from build123d import *

# Parameters (mm, degrees)
VERRUNDUNG1_R = 0.5


with BuildPart() as part:
    # Skizze1 → Rotation1 (revolve)
    with BuildSketch(Plane.XY, mode=Mode.PRIVATE) as rotation1_sk:
        Polygon((20, 0), (21.65, 0), (21.65, 0.5), (24.525, 0.5), (24.525, 0), (26, 0), (26, 7), (24.525, 7), (24.525, 6.5), (21.65, 6.5), (21.65, 7), (20, 7), align=None)
    revolve(rotation1_sk.sketch.rotate(Axis((0, 0, 0), (0, 1, 0)), 90), axis=Axis((0, 0, 0), (0, 1, 0)))

    # Verrundung1
    verrundung1_edges = [part.edges().sort_by_distance(p)[0] for p in [
        (0, 7, 26),
        (0, 0, 26),
        (0, 7, 20),
    ]]
    fillet(verrundung1_edges, radius=VERRUNDUNG1_R)


solid = part.part
Part model, mm, in its own coordinate system. A direction names the side the tool comes from. Coordinates: 2 decimals unless noted, no trailing zeros. Loops run counter-clockwise (first coordinate to the right, second up) from the corner with the lowest first, then second, coordinate; pieces in that order, holes last. Notation, with made-up numbers: (16, 62) -> (56, 62) arc R20 ccw to (56, 86) -> close; hole circle Ø11 at (16.25, -10.5). An arc over 180 degrees is marked (long way). Use a Markdown table: item, result. Add a question column.
Item 1: Which spindle directions (+Z, -Z, +X, -X, +Y, -Y) get a long thin tool onto all of the face, cutting with end or side? Do faces 1 (the flat face through (22, 6.5, 0)), 2 (the flat face through (19.1, 7, -7.9)), 3 (the cylindrical face through (21.758, 0.246, -11.317)). Say none if no direction does.
Item 2: Flat gauge pins, fed straight in: P1, Ø12, axis at x = 16, z = 18, coming from the +Y side; P2, Ø1.5, axis at x = 15, y = 6, coming from the -Z side; P3, Ø2, axis at y = 5.5, z = 0.5, coming from the +X side; P4, Ø3, axis at y = 4.5, z = 4.5, coming from the -X side. Where does each tip first touch, or does it go through?
Item 3: Band-saw the part on C-C on y = 5.75. Write the cut outline in (x, z).
Item 4: Pull direction Z, two halves, no side cores. Call faces 4 (the cylindrical face through (-0.88, 3.2, 19.98)), 5 (the cylindrical face through (15.821, 3.542, 20.633)), 6 (the flat face through (-13, 0, -21)): +Z half, -Z half, draft (parallel to the pull), parting line (faces both ways), or undercut.
Item 5: Probe probe 1 along X at (y, z) = (1.75, 0); probe 2 along Z at (x, y) = (0.5, 5.75); probe 3 along Y at (x, z) = (-20, 10). List the from-to ranges inside material, lowest first.
Geometry says:
| question | item | result |
|---|---|---|
| 1 | face 1 | +Y |
| 1 | face 2 | +Z, -Z, +X, -X, +Y |
| 1 | face 3 | -Y |
| 2 | P1 | y = 7 |
| 2 | P2 | z = -21.75 |
| 2 | P3 | x = 26 |
| 2 | P4 | x = -25.83 |
| 3 | outline | circle Ø52 at (0, 0); hole circle Ø40 at (0, 0) |
| 4 | face 4 | undercut |
| 4 | face 5 | parting line |
| 4 | face 6 | draft |
| 5 | probe 1 | -26 to -20, 20 to 26 |
| 5 | probe 2 | -26 to -19.99, 19.99 to 26 |
| 5 | probe 3 | 0.5 to 6.5 |
